Check sheet for the modelled part. Datum: model origin and axes. Units: mm. Face numbers are marked on the shaded views. A direction names the side the tool comes from. Give positions to 0.01 mm unless a question says otherwise; leave off trailing zeros. Order: outer loops, then holes, each group sorted by start corner. A loop starts at its lowest first (then second) coordinate and runs counter-clockwise, first axis right, second up.
Item 1: Release check for a two-part mould opening along X. For the marked faces 1, 2, 3 and 4 record: released by +X, released by -X, zero draft, split by the parting line, or undercut.
Item 2: Sectioned sample at D-D on z = -5.75. Record the boundary of the cut face in (x, y).
Item 3: Material ranges on line 1 along X through (y, z) = (15.5, -11); line 2 along Z through (x, y) = (17.5, 9.5); line 3 along Y through (x, z) = (0, -4.75), recorded low to high.
Item 4: Sectioned sample at B-B on z = 6.5. Record the boundary of the cut face in (x, y).
Item 5: Gauge pin test, flat ends, axial feed: P1, Ø4, axis at y = 3, z = -1, coming from the +X side; P2, Ø1, axis at y = -3.5, z = 1, coming from the +X side; P3, Ø8.5, axis at x = -10.5, z = 9, coming from the -Y side; P4, Ø4.5, axis at x = -12.75, y = -15.2, coming from the -Z side. Record the tip position at first contact, or that the pin passes through.
Item 6: Sectioned sample at A-A on x = 0. Record the boundary of the cut face in (y, z).
Item 7: Access from +Z, -Z, +X, -X, +Y, -Y to the whole of each face (thin tool, end or side, straight path). Record for the marked faces 5, 6, 7, 8 and 9.
Item 8: Sectioned sample at C-C on z = -10.5. Record the boundary of the cut face in (x, y).
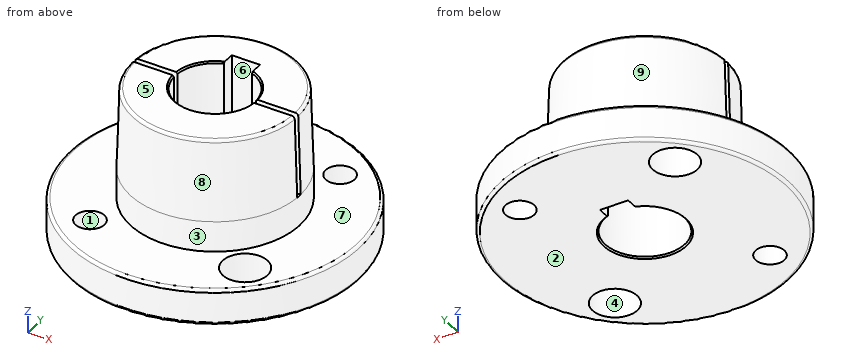
from build123d import *

# Parameters (mm, degrees)
FILLET1_R                        = 0.508
FILLET2_R                        = 0.508
CHAMFER1_SIZE                    = 0.254
SKETCH19_R                       = 2.54
THREADED_HOLES_1_DEPTH           = 42.03464937
SKETCH22_R                       = 3.937
CLEARANCE_HOLES_DEPTH            = 42.03464937
CLEARANCE_HOLES_CIRPATTERN_COUNT = 2
SKETCH23_W                       = 5
SKETCH23_H                       = 2.3
CUT_EXTRUDE1_DEPTH               = 45.453345531
CUT_EXTRUDE2_START               = -14.4526
SKETCH24_W                       = 29.7688
SKETCH24_H                       = 1
CUT_EXTRUDE2_DEPTH               = 14.4526


with BuildPart() as part:
    # Sketch1 → Revolve1 (revolve)
    with BuildSketch(Plane(origin=(0, 0, 0), x_dir=(0, 0, -1), z_dir=(1, 0, 0)), mode=Mode.PRIVATE) as revolve1_sk:
        Polygon((-13.0937, 7), (-13.0937, 14.432756404), (1.3589, 14.8844), (6.7437, 14.8844), (6.7437, 25.4), (13.0937, 25.4), (13.0937, 7), align=None)
    revolve(revolve1_sk.sketch.rotate(Axis((0, 0, 13.0937), (0, 0, -1)), 90), axis=Axis((0, 0, 13.0937), (0, 0, -1)))

    # Fillet1
    fillet1_edges = [part.edges().sort_by_distance(p)[0] for p in [
        (-25.4, 0, -13.0937),
        (-25.4, 0, -6.7437),
    ]]
    fillet(fillet1_edges, radius=FILLET1_R)

    # Fillet2
    fillet2_edges = [part.edges().sort_by_distance(p)[0] for p in [
        (-14.432756404, 0, 13.0937),
    ]]
    fillet(fillet2_edges, radius=FILLET2_R)

    # Chamfer1
    chamfer1_edges = [part.edges().sort_by_distance(p)[0] for p in [
        (-7, 0, -13.0937),
        (-7, 0, 13.0937),
    ]]
    chamfer(chamfer1_edges, length=CHAMFER1_SIZE)

    # Sketch19 → Threaded holes 1 (cut, through all)
    with BuildSketch(Plane.XY.offset(-6.7437)):
        with Locations((12.751234928, 15.196330036)):
            Circle(SKETCH19_R)
        with Locations((-12.751234928, -15.196330036)):
            Circle(SKETCH19_R)
    extrude(amount=-THREADED_HOLES_1_DEPTH, mode=Mode.SUBTRACT)

    # Sketch22 → Clearance holes (cut, through all)
    with BuildSketch(Plane.XY.offset(-6.7437)):
        with Locations((-14.027160061, 14.027160061)):
            Circle(SKETCH22_R)
    clearance_holes = extrude(amount=-CLEARANCE_HOLES_DEPTH, mode=Mode.SUBTRACT)

    # Clearance holes CirPattern: Clearance holes ×2 about axis
    clearance_holes_cirpattern_axis = Axis((0, 0, 0), (0, 0, 1))
    for i in range(1, CLEARANCE_HOLES_CIRPATTERN_COUNT):
        add(clearance_holes.rotate(clearance_holes_cirpattern_axis, i * 360 / CLEARANCE_HOLES_CIRPATTERN_COUNT), mode=Mode.SUBTRACT)

    # Sketch23 → Cut-Extrude1 (cut, through all)
    with BuildSketch(Plane.XY.offset(13.0937)):
        with Locations((0, 7.688348415)):
            Rectangle(SKETCH23_W, SKETCH23_H)
    extrude(amount=-CUT_EXTRUDE1_DEPTH, mode=Mode.SUBTRACT)

    # Sketch24 → Cut-Extrude2 (cut)
    with BuildSketch(Plane.XY.offset(13.0937).offset(CUT_EXTRUDE2_START)):
        Rectangle(SKETCH24_W, SKETCH24_H)
    extrude(amount=CUT_EXTRUDE2_DEPTH, mode=Mode.SUBTRACT)


solid = part.part
Report:
1. face 1: undercut
1. face 2: zero draft
1. face 3: split by the parting line
1. face 4: undercut
2. outline: circle Ø29.77 at (0, 0); hole (-2.5, 6.54) arc R7 ccw (long way) to (2.5, 6.54) - (2.5, 8.84) - (-2.5, 8.84) - close
3. line 1: x = -20.12 to -17.68, -10.38 to 10.23, 15.27 to 20.12
3. line 2: z = -13.09 to -6.74
3. line 3: y = -14.88 to -7, 8.84 to 14.88
4. outline: (-14.63, -0.5) arc R14.64 ccw to (14.63, -0.5) - (6.98, -0.5) arc R7 cw to (-6.98, -0.5) - close; (-14.63, 0.5) - (-6.98, 0.5) arc R7 cw to (-2.5, 6.54) - (-2.5, 8.84) - (2.5, 8.84) - (2.5, 6.54) arc R7 cw to (6.98, 0.5) - (14.63, 0.5) arc R14.64 ccw to start
5. P1: stops at x = 14.85
5. P2: stops at x = 14.5
5. P3: stops at y = -13.16
5. P4: passes through
6. outline: (-25.4, -12.59) arc R0.51 ccw to (-24.89, -13.09) - (-7.25, -13.09) - (-7, -12.84) - (-7, 12.84) - (-7.25, 13.09) - (-13.94, 13.09) arc R0.51 ccw to (-14.45, 12.6) - (-14.88, -1.36) - (-14.88, -6.74) - (-24.89, -6.74) arc R0.51 ccw to (-25.4, -7.25) - close; (8.84, -13.09) - (24.89, -13.09) arc R0.51 ccw to (25.4, -12.59) - (25.4, -7.25) arc R0.51 ccw to (24.89, -6.74) - (14.88, -6.74) - (14.88, -1.36) - (14.45, 12.6) arc R0.51 ccw to (13.94, 13.09) - (8.84, 13.09) - close
7. face 5: +Z, +X, -X, +Y, -Y
7. face 6: +Z, -Z
7. face 7: +Z
7. face 8: +Z, -Y
7. face 9: +Z, +Y
8. outline: circle Ø50.8 at (0, 0); hole circle Ø7.87 at (-14.03, 14.03); hole circle Ø5.08 at (-12.75, -15.2); hole (-2.5, 6.54) arc R7 ccw (long way) to (2.5, 6.54) - (2.5, 8.84) - (-2.5, 8.84) - close; hole circle Ø7.87 at (14.03, -14.03); hole circle Ø5.08 at (12.75, 15.2)
